The listing builds one solid part. Answer for the finished solid, in the listing's coordinates (mm). A direction names the side the tool comes from. Round coordinates to 2 decimals unless told otherwise and drop trailing zeros. Order: outer loops, then holes, each group sorted by start corner. A loop starts at its lowest first (then second) coordinate and runs counter-clockwise, first axis right, second up. Notation, with made-up numbers: M 40,79 L 55,79 A15 cw 55,91 Z; hole C -11,69.25 d4. An arc over 180 degrees is marked long. Write item = value, one per line. Start each with the question number.
(1) Straight lines are drawn through the part: probe 1 along Z at (x, y) = (149.5, 24.5); probe 2 along X at (y, z) = (100.5, 1030); probe 3 along Z at (x, y) = (-117, -18). For each, find the intervals that lie inside material, in ascending order. Write a range as from..to.
(2) Each of these flat-tipped pins is pushed along its axis until it touches: pin 1 (2 mm diameter, centred on x = -43, z = 245.5, fed in from +Y); pin 2 (8 mm diameter, centred on x = -35, y = -15, fed in from -Z); pin 3 (1.5 mm diameter, centred on x = 103.5, z = 870, fed in from -Y); pin 4 (1 mm diameter, centred on x = -3, y = 64, fed in from +Z). Where does it stop, or does it pass through?
(3) A cutting plane is placed at B-B, the plane x = 0. Determine the outline of the cut face in (y, z), and give its area (3 significant figures).
(4) A cutting plane is placed at C-C, the plane z = 427. Determine the outline of the cut face in (x, y).
(5) For a pull along X with two mould halves and no side action, classify faces 4 (the face through (169.59, 53.41, 989.18)), 5 (the face through (-114.83, -65.07, 1023.33)), 6 (the face through (1, 1, 0)) as released by +X, released by -X, zero draft, split by the parting line, or undercut.
(6) A cutting plane is placed at A-A, the plane z = 1015.5. Determine the outline of the cut face in (x, y).
(7) Which of the six approach directions +Z, -Z, +X, -X, +Y, -Y give full straight-line access (tool end or side, diameter ignored) to faces 1 (the face through (22.025, -99.184, 450.723)), 2 (the face through (1, 131.982, 1023)), 3 (the face through (27, 133, 1092.2))?
from build123d import *

# Parameters (mm, degrees)
SKETCH1_W           = 177.8
SKETCH1_H           = 203.2
SKETCH2_R           = 101.6
BOSS_EXTRUDE1_DEPTH = 889
CUT_EXTRUDE1_DEPTH  = 139.7


with BuildPart() as part:
    # Sketch1 → Revolve1 (revolve)
    with BuildSketch(Plane(origin=(0, 0, 0), x_dir=(1, 0, 0), z_dir=(0, 1, 0))):
        with Locations((88.9, -990.6)):
            Rectangle(SKETCH1_W, SKETCH1_H)
    revolve(axis=Axis((0, 0, 889), (0, 0, 1)))

    # Sketch2 → Boss-Extrude1 (add)
    with BuildSketch(Plane(origin=(0, 0, 889), x_dir=(-1, 0, 0), z_dir=(0, 0, -1))):
        Circle(SKETCH2_R)
    extrude(amount=BOSS_EXTRUDE1_DEPTH)

    # Sketch3 → Cut-Extrude1 (cut)
    with BuildSketch(Plane.XY.offset(1092.2)):
        Polygon((-152.4, 0), (-76.2, -131.982271537), (76.2, -131.982271537), (152.4, 0), (76.2, 131.982271537), (-76.2, 131.982271537), align=None)
    extrude(amount=-CUT_EXTRUDE1_DEPTH, mode=Mode.SUBTRACT)


solid = part.part
Reported:
q1.probe_1 = 889..1092.2
q1.probe_2 = -146.67..-94.38, 94.38..146.67
q1.probe_3 = 889..952.5
q2.pin_1 = 92.51
q2.pin_2 = 0
q2.pin_3 = through
q2.pin_4 = 952.5
q3.outline = M -177.8,889 L -101.6,889 L -101.6,0 L 101.6,0 L 101.6,889 L 177.8,889 L 177.8,1092.2 L 131.98,1092.2 L 131.98,952.5 L -131.98,952.5 L -131.98,1092.2 L -177.8,1092.2 Z
q3.area = 216,000 mm²
q4.outline = C 0,0 d203.2
q5.face_4 = split by the parting line
q5.face_5 = undercut
q5.face_6 = zero draft
q6.outline = C 0,0 d355.6; hole M -152.4,0 L -76.2,-131.98 L 76.2,-131.98 L 152.4,0 L 76.2,131.98 L -76.2,131.98 Z
q7.face_1 = -Z
q7.face_2 = +Z
q7.face_3 = +Z, +X, -X, +Y, -Y
